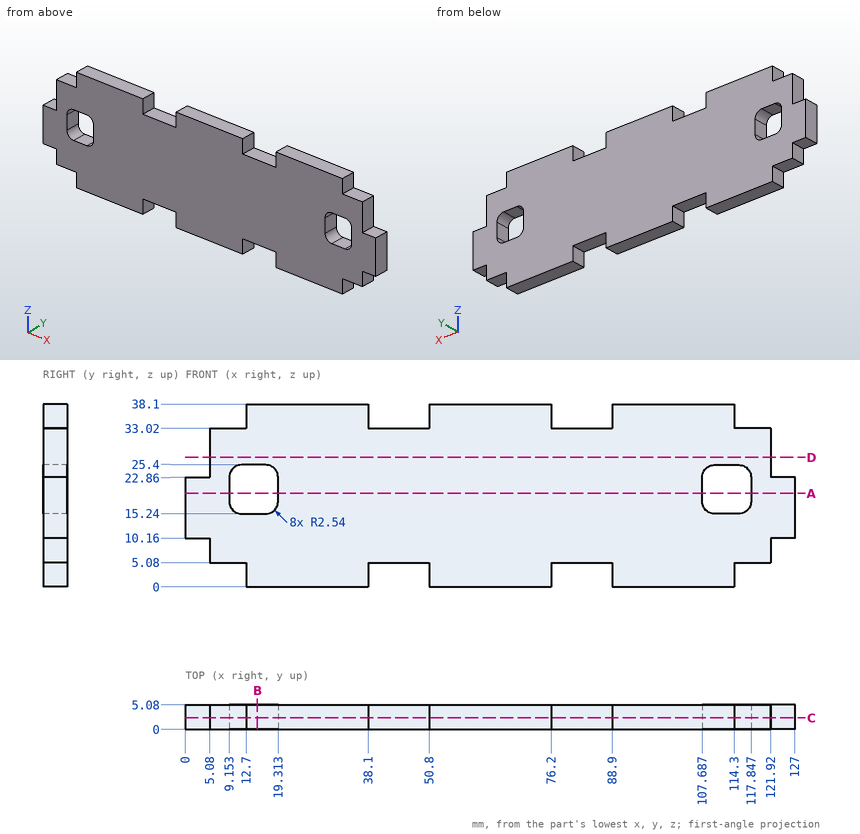
Design review of the part shown in the three views and the two pictorial views. Dimensions are in mm from the part's minimum x, y and z. Coordinates: 2 decimals unless noted, no trailing zeros. Write each loop counter-clockwise with the first axis right and the second up, starting at its lowest first coordinate (ties: lowest second). Pieces come first, ordered by that corner, then holes. Notation, with made-up numbers: (-38.75, -28.75) - (-16.75, -28.75) arc R31 ccw to (-16.75, -4.75) - close; hole circle Ø2 at (-34.5, 39). An arc over 180 degrees is marked (long way). Write item = value, one per line.
(1) Consider section B-B, the plane x = 15. Give the boundary of the cut face in (y, z), then the cut area to 3 significant figures.
Result sheet:
outline = (0, 0) - (5.08, 0) - (5.08, 15.24) - (0, 15.24) - close; (0, 25.4) - (5.08, 25.4) - (5.08, 38.1) - (0, 38.1) - close
area = 142 mm^2
(2) Consider section C-C, the plane y = 2.35. State how many separate pieces and enclosed holes the cut face has, then the cut area to 3 significant figures.
Result sheet:
separate_pieces = 1
enclosed_holes = 2
area = 3,970 mm^2
(3) Consider section D-D, the plane z = 27. Give the boundary of the cut face in (x, y).
Result sheet:
outline = (5.08, 0) - (121.92, 0) - (121.92, 5.08) - (5.08, 5.08) - close
(4) Consider section A-A, the plane z = 19.5. Give the boundary of the cut face in (x, y).
Result sheet:
outline = (0, 0) - (9.15, 0) - (9.15, 5.08) - (0, 5.08) - close; (19.31, 0) - (107.69, 0) - (107.69, 5.08) - (19.31, 5.08) - close; (117.85, 0) - (127, 0) - (127, 5.08) - (117.85, 5.08) - close
(5) For P1, Ø2.5, axis at y = 2.5, z = 34.5, coming from the -X side; P2, Ø1.5, axis at x = 46, y = 2.5, coming from the +Z side; P3, Ø2, axis at y = 2, z = 18, coming from the -X side; P4, Ø1.5, axis at y = 3, z = 1.5, coming from the +X side, all flat-tipped, find the tip position at first contact; note any pin that passes through.
Result sheet:
P1 = 12.7
P2 = 33.02
P3 = 0
P4 = 114.3
(6) For line 1 (X direction, y = 1.4, z = 21.5); line 2 (X direction, y = 4.35, z = 35.5); line 3 (X direction, y = 2.95, z = 7), list the stretches that pass through material, from the lowest coordinate up. Write a range as [from, to].
Result sheet:
line_1 = [0, 9.15], [19.31, 107.69], [117.85, 127]
line_2 = [12.7, 38.1], [50.8, 76.2], [88.9, 114.3]
line_3 = [5.08, 121.92]
